Autodesk Inventor part; units mm, degrees
ref_plane "YZ Plane" through (0, 0, 0) normal (1, 0, 0) x (0, 1, 0)
ref_plane "XZ Plane" through (0, 0, 0) normal (0, 1, 0) x (-1, 0, 0)
ref_plane "XY Plane" through (0, 0, 0) normal (0, 0, 1) x (1, 0, 0)
sketch "Sketch1" plane through (0, 0, 0) normal (0, 0, 1) x (1, 0, 0)
  line L0 (-3.25, 6.4) -> (3.25, 6.4)
  line L1 (3.25, 6.4) -> (3.25, -6.4)
  line L2 (3.25, -6.4) -> (-3.25, -6.4)
  line L3 (-3.25, -6.4) -> (-3.25, 6.4)
  line L4 (-3.25, 6.4) -> (3.25, -6.4) construction
  line L5 (3.25, 6.4) -> (-3.25, -6.4) construction
  line L6 (3.25, -6.4) -> (3.25, 6.4)
  line L7 (3.25, 6.4) -> (6.25, 6.4)
  line L8 (6.25, 6.4) -> (6.25, -11.6)
  line L9 (6.25, -11.6) -> (3.25, -11.6)
  line L10 (3.25, -11.6) -> (3.25, 6.4)
  line L11 (-3.25, 6.4) -> (-6.55, 6.4)
  line L12 (-6.55, 6.4) -> (-6.55, -6.4)
  line L13 (-6.55, -6.4) -> (-3.25, -6.4)
  line L14 (-3.25, -6.4) -> (-3.25, 6.4)
  line L15 (3.25, 0) -> (-3.25, 0) construction
  point P0 (0, 0)
  point P1 (-1.75, -3.25)
  point P2 (-1.75, 3.25)
  dimension "d0" = 6.5
  dimension "d5" = 12.8
  dimension "d6" = 18
  dimension "d7" = 9.5
  dimension "d8" = 3.3
  dimension "d13" = 6.5
  dimension "d14" = 1.5
extrude "Extrusion1" add sketch "Sketch1" along normal blind 5.7
hole "Hole1" at (-1.75, -3.25, 0) at (-1.75, 3.25, 0) direction (0, 0, 1) diameter 2.1 end through all
properties part number "Endstop"
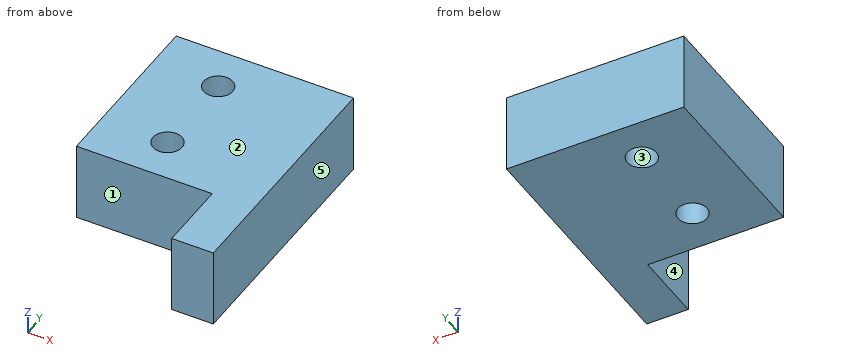
Work out the finished part from the listing and answer in its coordinate system (mm). Face numbers are marked on the shaded views. A direction names the side the tool comes from. Give positions to 0.01 mm unless a question says otherwise; leave off trailing zeros. Loops run counter-clockwise (first coordinate to the right, second up) from the corner with the lowest first, then second, coordinate; pieces in that order, holes last. Notation, with made-up numbers: (73, 6.25) - (118, 6.25) arc R22 ccw to (118, 41.25) - close; hole circle Ø3 at (-1, 56.5). An arc over 180 degrees is marked (long way). Answer in a Markdown table with one row per item.
(1) For a pull along Y with two mould halves and no side action, classify the marked faces 1, 2 and 3 as pulls with the +Y half, pulls with the -Y half, needs draft (parallel to the pull), parting line crosses it, or undercut.
Results list:
| item | result |
|---|---|
| face 1 | pulls with the -Y half |
| face 2 | needs draft |
| face 3 | undercut |
(2) Flat-ended cylindrical pins translate along their axes: pin 1 Ø1.5 at (x, z) = (-2.5, 1.5) entering from -Y; pin 2 Ø1 at (x, y) = (1.5, -9.5) entering from +Z; pin 3 Ø1.6 at (y, z) = (-9.5, 1.5) entering from -X. Find the tip coordinate at first contact, or state that the pin passes through.
Results list:
| item | result |
|---|---|
| pin 1 | stops at y = -6.4 |
| pin 2 | passes through |
| pin 3 | stops at x = 3.25 |
(3) Section D-D (y = -8.75) is taken. Give the vertices of the cut face in (x, z).
Results list:
| item | result |
|---|---|
| outline | (3.25, 0) - (6.25, 0) - (6.25, 5.7) - (3.25, 5.7) - close |
(4) Section B-B (x = -1.75) is taken. Give the vertices of the cut face in (y, z).
Results list:
| item | result |
|---|---|
| outline | (-6.4, 0) - (-4.3, 0) - (-4.3, 5.7) - (-6.4, 5.7) - close; (-2.2, 0) - (2.2, 0) - (2.2, 5.7) - (-2.2, 5.7) - close; (4.3, 0) - (6.4, 0) - (6.4, 5.7) - (4.3, 5.7) - close |
(5) A tool of negligible diameter and unlimited length cuts with its end or side. For the marked faces 4 and 5, from which of +Z, -Z, +X, -X, +Y, -Y can it reach the whole face along a straight path? Write none if from no direction.
Results list:
| item | result |
|---|---|
| face 4 | +Z, -Z, -X, -Y |
| face 5 | +Z, -Z, +X, +Y, -Y |
(6) Section A-A (y = -3.25) is taken. Give the vertices of the cut face in (x, z).
Results list:
| item | result |
|---|---|
| outline | (-6.55, 0) - (-2.8, 0) - (-2.8, 5.7) - (-6.55, 5.7) - close; (-0.7, 0) - (6.25, 0) - (6.25, 5.7) - (-0.7, 5.7) - close |
(7) Section C-C (z = 1.15) is taken. Give the vertices of the cut face in (x, y), and give its area (3 significant figures).
Results list:
| item | result |
|---|---|
| outline | (-6.55, -6.4) - (3.25, -6.4) - (3.25, -11.6) - (6.25, -11.6) - (6.25, 6.4) - (-6.55, 6.4) - close; hole circle Ø2.1 at (-1.75, -3.25); hole circle Ø2.1 at (-1.75, 3.25) |
| area | 173 mm² |
(8) Consider L1, parallel to X at y = -3.25, z = 2.3; L2, parallel to Y at x = -1, z = 3.1; L3, parallel to Y at x = 0.5, z = 1.45. Determine where each line is inside the solid, lowest interval first. Write a range as [from, to].
Results list:
| item | result |
|---|---|
| L1 | x = [-6.55, -2.8], [-0.7, 6.25] |
| L2 | y = [-6.4, -3.98], [-2.52, 2.52], [3.98, 6.4] |
| L3 | y = [-6.4, 6.4] |
